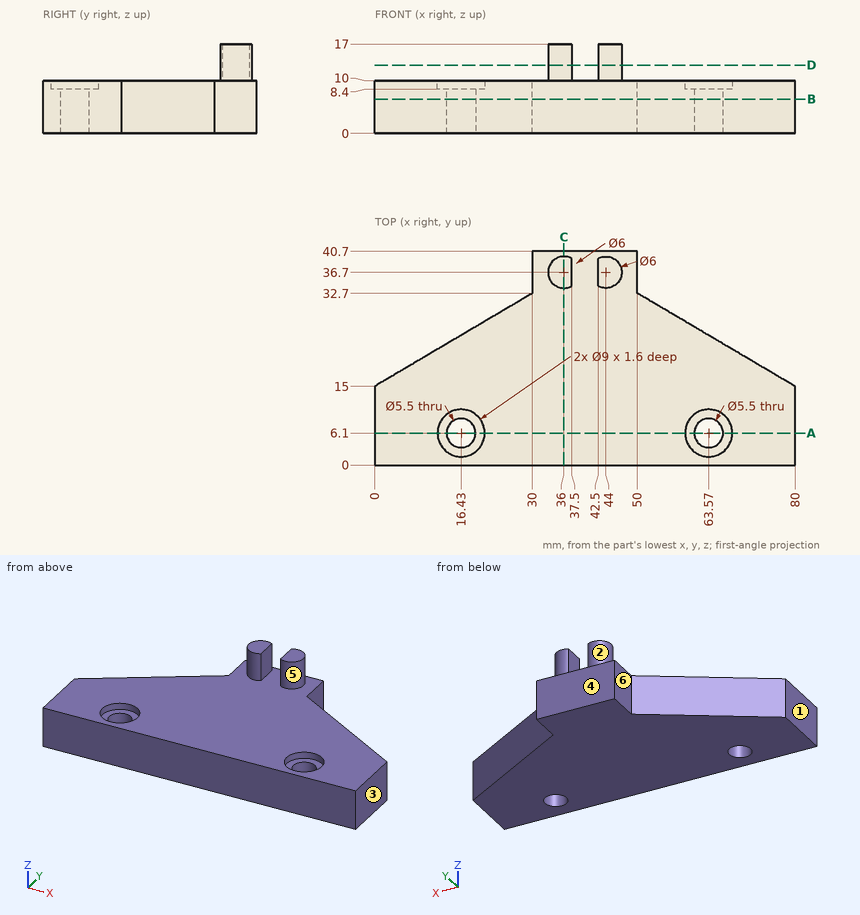
Geometry: see drawing. Coordinates: mm, zero at the bounding-box minimum. A direction names the side the tool comes from. Give positions to 0.01 mm unless a question says otherwise; leave off trailing zeros. Loops run counter-clockwise (first coordinate to the right, second up) from the corner with the lowest first, then second, coordinate; pieces in that order, holes last. Notation, with made-up numbers: (-5.5, 29.25) - (21.5, 29.25) arc R12 ccw to (21.5, 44.25) - close; hole circle Ø4 at (-6.5, 72.5). An arc over 180 degrees is marked (long way). Use CSV: the item, a comma, the result in double quotes.
1) Cut plane D-D (z = 13). Output: boundary loops of the cut face in (x, y).
Worked out:
outline,"(37.5, 34.1) - (37.5, 39.3) arc R3 ccw (long way) to start; (42.5, 34.1) arc R3 ccw (long way) to (42.5, 39.3) - close"
2) Cut plane C-C (x = 36). Output: boundary loops of the cut face in (y, z), and give its area (3 significant figures).
Worked out:
outline,"(0, 0) - (40.7, 0) - (40.7, 10) - (39.7, 10) - (39.7, 17) - (33.7, 17) - (33.7, 10) - (0, 10) - close"
area,"449 mm^2"
3) Line query: line 1 (Z direction, x = 16.5, y = 23); line 2 (X direction, y = 6.5, z = 2); line 3 (X direction, y = 36, z = 9.75). Output: solid intervals per line, ascending.
Worked out:
line 1,"z = 0 to 10"
line 2,"x = 0 to 13.71, 19.15 to 60.85, 66.29 to 80"
line 3,"x = 30 to 50"
4) Set-up query: the marked faces 4, 5 and 6. Return all of +Z, -Z, +X, -X, +Y, -Y with unobstructed straight access to the full face (end or side cutting, diameter ignored); none if empty.
Worked out:
face 4,"+Z, -Z, +X, -X, +Y"
face 5,"+Z"
face 6,"+Z, -Z, -X, +Y"
5) Pin query (flat end, axial travel): P1, Ø6, axis at x = 68, z = 10, coming from the -Y side; P2, Ø20.5, axis at x = 45.5, y = 20.5, coming from the +Z side; P3, Ø4, axis at x = 46, z = 14, coming from the +Y side; P4, Ø9, axis at y = 35.5, z = 3.5, coming from the +X side. Return the tip coordinate at first contact, or that it passes through.
Worked out:
P1,"stops at y = 0"
P2,"stops at z = 10"
P3,"stops at y = 39.7"
P4,"stops at x = 52.88"
6) Cut plane B-B (z = 6.5). Output: boundary loops of the cut face in (x, y), and give its area (3 significant figures).
Worked out:
outline,"(0, 0) - (80, 0) - (80, 15) - (50, 32.7) - (50, 40.7) - (30, 40.7) - (30, 32.7) - (0, 15) - close; hole circle Ø5.5 at (16.43, 6.1); hole circle Ø5.5 at (63.57, 6.1)"
area,"2,200 mm^2"
7) Mould query, pull axis X, two halves, no side actions, for the marked faces 1, 2 and 3. Classes: +X half, -X half, draft (parallel to the pull), parting line (faces both ways), or undercut.
Worked out:
face 1,"-X half"
face 2,"undercut"
face 3,"+X half"
8) Cut plane A-A (y = 6.1). Output: boundary loops of the cut face in (x, z), and give its area (3 significant figures).
Worked out:
outline,"(0, 0) - (13.68, 0) - (13.68, 8.4) - (11.93, 8.4) - (11.93, 10) - (0, 10) - close; (19.18, 0) - (60.82, 0) - (60.82, 8.4) - (59.07, 8.4) - (59.07, 10) - (20.93, 10) - (20.93, 8.4) - (19.18, 8.4) - close; (66.32, 0) - (80, 0) - (80, 10) - (68.07, 10) - (68.07, 8.4) - (66.32, 8.4) - close"
area,"679 mm^2"
